Verification items for the finished model (mm, model axes). A direction names the side the tool comes from. Round coordinates to 2 decimals unless told otherwise and drop trailing zeros. Write each loop counter-clockwise with the first axis right and the second up, starting at its lowest first coordinate (ties: lowest second). Pieces come first, ordered by that corner, then holes. Notation, with made-up numbers: (-19.75, -4) - (35.25, -4) arc R12 cw to (35.25, 14) - close; hole circle Ø5 at (-21.5, -14). An arc over 180 degrees is marked (long way). Answer as a JSON object with one key per item and string values. Group by question number.
1) Mould release check, pull along X, two halves, no side actions. Record for faces 4 (the flat face through (6, 11, 10)), 5 (the cylindrical face through (-13.355, 6.782, 15.227)), 6 (the flat face through (0, 8, 2)): +X half, -X half, draft (parallel to the pull), parting line (faces both ways), or undercut.
2) Section check B-B (z = 67). Enter the section's corners in (x, y).
3) Thickness scan on line 1 (X direction, y = 7.25, z = 238.5); line 2 (X direction, y = 8.8, z = 0); line 3 (Z direction, x = 0.5, y = 10.75). Record the ranges inside material, lowest first.
4) Section check A-A (y = 5.5). State how many separate pieces and enclosed holes the cut face has, then the cut area to 3 significant figures.
5) Go/stop test with flat-tipped pins: pin 1 Ø2 at (x, z) = (6.06, -3.5) entering from +Y; pin 2 Ø3 at (x, y) = (2.5, 6) entering from +Z; pin 3 Ø17.5 at (x, z) = (-5.5, 184.5) entering from +Y; pin 4 Ø5 at (x, z) = (-7.36, 4.25) entering from +Y. Record where each tip stops, or that it passes through.
6) Set-up check for faces 1 (the flat face through (-8.4, 7, 247.8)), 2 (the cylindrical face through (-13.18, 9.99, -2.93)), 3 (the flat face through (12.5, 7, 140)): record each of +Z, -Z, +X, -X, +Y, -Y from which the full face is reachable in a straight line by a thin tool's end or side.
```python
from build123d import *
from build123d.topology import SkipClean

# Parameters (mm, degrees)
EXTRUDE_1_DEPTH              = 9
SKETCH_3_R                   = 13.5
EXTRUDE_2_DEPTH              = 2
SKETCH_4_R                   = 13.5
EXTRUDE_3_DEPTH              = 3
SKETCH_5_R                   = 9.5
CUT_EXTRUDE_2_DEPTH          = 274.324898244
HOLE_WIZARD_M3_1_D           = 3.4
HOLE_WIZARD_M3_1_CBORE_D     = 6.5
HOLE_WIZARD_M3_1_CBORE_DEPTH = 3.4
PATTERN_CIRCULAR_1_COUNT     = 3
SKETCH_11_R                  = 12.5
SKETCH_11_R_2                = 3.25
EXTRUDE_4_DEPTH              = 7
SKETCH_13_R                  = 11.5
CUT_EXTRUDE_3_DEPTH          = 3
FILLET_1_R                   = 40
SKETCH_26_W                  = 65.136073631
SKETCH_26_H                  = 24.89875822
CUT_EXTRUDE_5_DEPTH          = 1111
SKETCH_28_R                  = 9.5
SKETCH_28_R_2                = 8.5
EXTRUDE_5_DEPTH              = 2
HOLE_WIZARD_M3_2_D           = 2.5
PATTERN_LINEAR_1_COUNT       = 3
PATTERN_LINEAR_1_PITCH       = 70
PATTERN_LINEAR_1_COUNT_DIR2  = 2
PATTERN_LINEAR_1_PITCH_DIR2  = 10
HOLE_WIZARD_M3_3_D           = 2.5
PATTERN_CIRCULAR_4_COUNT     = 6
SKETCH_44_R                  = 1.25
EXTRUDE_6_DEPTH              = 4.5
F_3_0MM_2_D                  = 3
F_3_0MM_2_DEPTH              = 5
F_3_0MM_2_TIP                = 0.901290929
PATTERN_CIRCULAR_5_COUNT     = 3


with BuildPart() as part:
    # Sketch 1 → Extrude 1 (new body)
    with BuildSketch(Plane(origin=(0, 0, 0), x_dir=(1, 0, 0), z_dir=(0, 1, 0))):
        with BuildLine():
            Line((-12.5, -260), (-12.5, -12.247448714))
            ThreePointArc((-12.5, -12.247448714), (0, 17.5), (12.5, -12.247448714))
            Line((12.5, -12.247448714), (12.5, -260))
            ThreePointArc((12.5, -260), (0, -272.5), (-12.5, -260))
        make_face()
    extrude(amount=EXTRUDE_1_DEPTH)

    # Sketch 3 → Extrude 2 (add)
    with BuildSketch(Plane(origin=(0, 9, 0), x_dir=(1, 0, 0), z_dir=(0, 1, 0))):
        with Locations(Location((0, 0, 0), (0, 0, 270))):
            Circle(SKETCH_3_R)
    extrude(amount=EXTRUDE_2_DEPTH)

    # Sketch 4 → Extrude 3 (add)
    with BuildSketch(Plane.XZ):
        with Locations(Location((0, 0, 0), (0, 0, 90))):
            Circle(SKETCH_4_R)
    extrude(amount=EXTRUDE_3_DEPTH)

    # Sketch 5 → Cut-Extrude 2 (cut, through all)
    with BuildSketch(Plane(origin=(0, 9, 0), x_dir=(1, 0, 0), z_dir=(0, 1, 0))):
        with Locations(Location((0, -250, 0), (0, 0, 270))):
            Circle(SKETCH_5_R)
    extrude(amount=-CUT_EXTRUDE_2_DEPTH, mode=Mode.SUBTRACT)

    # Hole Wizard M3 _ _ _ _ _ _1 (through all)
    with Locations(Plane(origin=(0, -3, 0), x_dir=(-1, 0, 0), z_dir=(0, -1, 0))):
        with Locations((0, -7)):
            hole_wizard_m3_1 = CounterBoreHole(HOLE_WIZARD_M3_1_D / 2, HOLE_WIZARD_M3_1_CBORE_D / 2, HOLE_WIZARD_M3_1_CBORE_DEPTH)

    # Pattern Circular 1: Hole Wizard M3 _ _ _ _ _ _1 ×3 about axis
    pattern_circular_1_axis = Axis((0, 0, 0), (0, 1, 0))
    for i in range(1, PATTERN_CIRCULAR_1_COUNT):
        add(hole_wizard_m3_1.rotate(pattern_circular_1_axis, i * 360 / PATTERN_CIRCULAR_1_COUNT), mode=Mode.SUBTRACT)

    # Sketch 11 → Extrude 4 (add)
    with SkipClean():  # the faces are left unmerged after this step: merging them gives an invalid solid
        with BuildSketch(Plane.XZ.offset(3)):
            with Locations(Location((0, 0, 0), (0, 0, 270))):
                Circle(SKETCH_11_R)
            with Locations(Location((6.062177826, -3.5, 0), (0, 0, 270))):
                Circle(SKETCH_11_R_2, mode=Mode.SUBTRACT)
            with Locations(Location((0, 7, 0), (0, 0, 270))):
                Circle(SKETCH_11_R_2, mode=Mode.SUBTRACT)
            with Locations(Location((-6.062177826, -3.5, 0), (0, 0, 270))):
                Circle(SKETCH_11_R_2, mode=Mode.SUBTRACT)
        extrude(amount=EXTRUDE_4_DEPTH)

    # Sketch 13 → Cut-Extrude 3 (cut)
    with SkipClean():  # the faces are left unmerged after this step: merging them gives an invalid solid
        with BuildSketch(Plane(origin=(0, 11, 0), x_dir=(1, 0, 0), z_dir=(0, 1, 0))):
            with Locations(Location((0, 0, 0), (0, 0, 270))):
                Circle(SKETCH_13_R)
        extrude(amount=-CUT_EXTRUDE_3_DEPTH, mode=Mode.SUBTRACT)

    # Fillet 1
    fillet_1_edges = [part.edges().sort_by_distance(p)[0] for p in [
        (12.5, 4.5, 12.247448714),
        (-12.5, 4.5, 12.247448714),
    ]]
    fillet(fillet_1_edges, radius=FILLET_1_R)

    # Sketch 26 → Cut-Extrude 5 (cut, symmetric)
    with BuildSketch(Plane.XY):
        with Locations((0.11753139, -7.94937911)):
            Rectangle(SKETCH_26_W, SKETCH_26_H)
    extrude(amount=CUT_EXTRUDE_5_DEPTH, both=True, mode=Mode.SUBTRACT)

    # Sketch 28 → Extrude 5 (add)
    with BuildSketch(Plane(origin=(0, 9, 0), x_dir=(1, 0, 0), z_dir=(0, 1, 0))):
        with Locations(Location((0, -250, 0), (0, 0, 270))):
            Circle(SKETCH_28_R)
        with Locations(Location((0, -250, 0), (0, 0, 270))):
            Circle(SKETCH_28_R_2, mode=Mode.SUBTRACT)
    extrude(amount=-EXTRUDE_5_DEPTH)

    # Hole Wizard M3 _ _ _ _2 (through all)
    with Locations(Plane(origin=(0, 4.5, 0), x_dir=(-1, 0, 0), z_dir=(0, -1, 0))):
        with Locations((5, -25)):
            hole_wizard_m3_2 = Hole(HOLE_WIZARD_M3_2_D / 2)

    # Pattern Linear 1: Hole Wizard M3 _ _ _ _2 3 × 2
    with Locations(*[(j * PATTERN_LINEAR_1_PITCH_DIR2, 0, i * PATTERN_LINEAR_1_PITCH) for i in range(PATTERN_LINEAR_1_COUNT) for j in range(PATTERN_LINEAR_1_COUNT_DIR2) if (i, j) != (0, 0)]):
        add(hole_wizard_m3_2, mode=Mode.SUBTRACT)

    # Hole Wizard M3 _ _ _ _3 (through all)
    with Locations(Plane(origin=(0, 4.5, 0), x_dir=(-1, 0, 0), z_dir=(0, -1, 0))):
        with Locations((6.75, -261.691342951)):
            hole_wizard_m3_3 = Hole(HOLE_WIZARD_M3_3_D / 2)

    # Pattern Circular 4: Hole Wizard M3 _ _ _ _3 ×6 about axis, 2 skipped
    pattern_circular_4_axis = Axis((0, 0, 250), (0, 1, 0))
    add([hole_wizard_m3_3.rotate(pattern_circular_4_axis, i * 360 / PATTERN_CIRCULAR_4_COUNT) for i in range(1, PATTERN_CIRCULAR_4_COUNT) if i not in (2, 5)], mode=Mode.SUBTRACT)

    # Sketch 44 → Extrude 6 (add)
    with BuildSketch(Plane.XZ.offset(-4.5)):
        with Locations((5, 25)):
            Circle(SKETCH_44_R)
        with Locations((-5, 25)):
            Circle(SKETCH_44_R)
    extrude(amount=-EXTRUDE_6_DEPTH)

    # 3.0mm _ _2
    with Locations(Plane(origin=(0, 4.5, 0), x_dir=(-1, 0, 0), z_dir=(0, -1, 0))):
        with Locations((0, 0)):
            Hole(F_3_0MM_2_D / 2, depth=F_3_0MM_2_DEPTH)
            with Locations((0, 0, -(F_3_0MM_2_DEPTH + F_3_0MM_2_TIP / 2))):  # 118° drill point
                Cone(0, F_3_0MM_2_D / 2, F_3_0MM_2_TIP, mode=Mode.SUBTRACT)

    # Sketch 50 → 3.0mm _ _3 (revolve, cut)
    with BuildSketch(Plane(origin=(0, 8, -8.5), x_dir=(0, 0, 1), z_dir=(1, 0, 0))):
        Polygon((0, 0), (0, 5.901290929), (1.5, 5), (1.5, 0), align=None)
    f_3_0mm_3 = revolve(axis=Axis((0, 14.35, -8.5), (0, -1, 0)), mode=Mode.SUBTRACT)

    # Pattern Circular 5: 3.0mm _ _3 ×3 about axis
    pattern_circular_5_axis = Axis((0, 0, 0), (0, 1, 0))
    for i in range(1, PATTERN_CIRCULAR_5_COUNT):
        add(f_3_0mm_3.rotate(pattern_circular_5_axis, i * 360 / PATTERN_CIRCULAR_5_COUNT), mode=Mode.SUBTRACT)


solid = part.part
```
Returned:
{
 "1": {"face 4": "draft", "face 5": "-X half", "face 6": "undercut"},
 "2": {"outline": "(-12.5, 4.5) - (12.5, 4.5) - (12.5, 9) - (-12.5, 9) - close"},
 "3": {"line 1": "-12.5 to -7.99, -5.51 to 5.51, 7.99 to 12.5", "line 2": "-17.5 to -11.5, 11.5 to 17.5", "line 3": "-13.49 to -11.49, 11.49 to 13.49"},
 "4": {"separate pieces": "1", "enclosed holes": "16", "area": "6,950 mm2"},
 "5": {"pin 1": "through", "pin 2": "z = 272.46", "pin 3": "y = 9", "pin 4": "y = 8"},
 "6": {"face 1": "-Y", "face 2": "+Y", "face 3": "+Z, +X, +Y, -Y"}
}
